from build123d import *

# Parameters (mm, degrees)
F0_R     = 20.8565821632
F1_DEPTH = 25.4


with BuildPart() as f1:
    # F0 (on Top) → F1 (new body)
    with BuildSketch(Plane.XY):
        with BuildLine():
            Line((-41.851490736, 0), (-138.5076195002, 0))
            Line((-138.5076195002, 0), (-116.6970655322, -86.8278518319))
            Line((-116.6970655322, -86.8278518319), (0, -86.8278518319))
            Line((0, -86.8278518319), (-17.9794709813, -49.5264602942))
            ThreePointArc((-17.9794709813, -49.5264602942), (-43.2116401305, -74.6403530851), (-75.7857334668, -60.2772609946))
            ThreePointArc((-75.7857334668, -60.2772609946), (-115.8407580084, -55.5523652684), (-79.8986506619, -37.2522409479))
            ThreePointArc((-79.8986506619, -37.2522409479), (-62.4846109467, -15.0805313011), (-34.2980027941, -15.6709622596))
            Line((-34.2980027941, -15.6709622596), (-41.851490736, 0))
        make_face()
        with BuildLine():
            ThreePointArc((-17.4199218149, -43.6096377671), (-21.9669745384, -27.2891046366), (-34.2980027941, -15.6709622596))
            Line((-34.2980027941, -15.6709622596), (-17.9794709813, -49.5264602942))
            ThreePointArc((-17.9794709813, -49.5264602942), (-17.5601204804, -46.5812486134), (-17.4199218149, -43.6096377671))
        make_face()
        with BuildLine():
            Line((-17.9794709813, -49.5264602942), (-34.2980027941, -15.6709622596))
            ThreePointArc((-34.2980027941, -15.6709622596), (-62.4846109467, -15.0805313011), (-79.8986506619, -37.2522409479))
            ThreePointArc((-79.8986506619, -37.2522409479), (-75.5491310736, -43.9810085097), (-74.0258815603, -51.8470332026))
            ThreePointArc((-74.0258815603, -51.8470332026), (-74.4705361025, -56.1530121668), (-75.7857334668, -60.2772609946))
            ThreePointArc((-75.7857334668, -60.2772609946), (-43.2116401305, -74.6403530851), (-17.9794709813, -49.5264602942))
        make_face()
        with Locations((-48.9827282727, -43.6096377671)):
            Circle(F0_R, mode=Mode.SUBTRACT)
    extrude(amount=F1_DEPTH)


solid = f1.part
The listing builds one solid part. Answer for the finished solid, in the listing's coordinates (mm). Give positions to 0.01 mm unless a question says otherwise; leave off trailing zeros. Order: outer loops, then holes, each group sorted by start corner. A loop starts at its lowest first (then second) coordinate and runs counter-clockwise, first axis right, second up. Notation, with made-up numbers: (57, 0.25) - (76, 0.25) arc R35 cw to (76, 33.25) - close; hole circle Ø11 at (-24.5, 17.25). An arc over 180 degrees is marked (long way). Use one line per item in the form item = value.
1) Consider probe 1 along X at (y, z) = (-50.5, 23.25); probe 2 along X at (y, z) = (-43, 19.5); probe 3 along Y at (x, z) = (-35, 11.5). Determine where each line is inside the solid, lowest interval first. Write a range as [from, to].
Verdict:
probe_1 = [-125.82, -116.13], [-74.07, -68.67], [-29.3, -17.51]
probe_2 = [-127.71, -114.22], [-75.97, -69.83], [-28.14, -17.43]
probe_3 = [-86.83, -59.08], [-28.13, -14.21]
2) Find section D-D on y = -36.5. Determine the outline of the cut face in (x, z), and give its area (3 significant figures).
Verdict:
outline = (-129.34, 0) - (-109.54, 0) - (-109.54, 25.4) - (-129.34, 25.4) - close; (-80.66, 0) - (-68.59, 0) - (-68.59, 25.4) - (-80.66, 25.4) - close; (-29.38, 0) - (-18.23, 0) - (-18.23, 25.4) - (-29.38, 25.4) - close
area = 1,090 mm^2
3) Find section A-A on y = -59.5. Determine the outline of the cut face in (x, z), and give its area (3 significant figures).
Verdict:
outline = (-123.56, 0) - (-114.73, 0) - (-114.73, 25.4) - (-123.56, 25.4) - close; (-75.46, 0) - (-62.49, 0) - (-62.49, 25.4) - (-75.46, 25.4) - close; (-35.47, 0) - (-13.17, 0) - (-13.17, 25.4) - (-35.47, 25.4) - close
area = 1,120 mm^2
4) Each of these flat-tipped pins is pushed along its axis until it touches: pin 1 (12 mm diameter, centred on x = -25, z = 16, fed in from +Y); pin 2 (6 mm diameter, centred on y = -41, z = 11, fed in from -X); pin 3 (1 mm diameter, centred on y = -23.5, z = 10, fed in from -X). Where does it stop, or does it pass through?
Verdict:
pin_1 = -17.67
pin_2 = -128.96
pin_3 = -132.73
5) Find section C-C on z = 20. Determine the outline of the cut face in (x, y).
Verdict:
outline = (-138.51, 0) - (-116.7, -86.83) - (0, -86.83) - (-17.98, -49.53) arc R31.56 ccw to (-34.3, -15.67) - (-41.85, 0) - close; hole circle Ø42.14 at (-95.1, -51.85); hole circle Ø41.71 at (-48.98, -43.61)
6) Find section B-B on x = -112. Determine the outline of the cut face in (y, z), and give its area (3 significant figures).
Verdict:
outline = (-86.83, 0) - (-64.43, 0) - (-64.43, 25.4) - (-86.83, 25.4) - close; (-39.26, 0) - (0, 0) - (0, 25.4) - (-39.26, 25.4) - close
area = 1,570 mm^2
7) The mould has two halves that part along Y. Classify faces 1 (the flat face through (-70, -43, 0)), 2 (the cylindrical face through (-37.77, -26.023, 12.522)), 3 (the flat face through (-90, 0, 13)): released by +Y, released by -Y, zero draft, split by the parting line, or undercut.
Verdict:
face_1 = zero draft
face_2 = undercut
face_3 = released by +Y
